Autodesk Inventor part; units mm, degrees
ref_plane "YZ Plane" through (0, 0, 0) normal (1, 0, 0) x (0, 1, 0)
ref_plane "XZ Plane" through (0, 0, 0) normal (0, 1, 0) x (-1, 0, 0)
ref_plane "XY Plane" through (0, 0, 0) normal (0, 0, 1) x (1, 0, 0)
sketch "Sketch1" plane through (0, 0, 0) normal (0, 1, 0) x (-1, 0, 0)
  circle A0 centre (0, 0) radius 13
  circle A1 centre (0, 0) radius 14.5
  dimension "d0" = 26
  dimension "d1" = 29
extrude "Extrusion1" add sketch "Sketch1" along normal blind 4
sketch "Sketch2" plane through (0, 0, 0) normal (0, -1, 0) x (1, 0, 0)
  circle A0 centre (0, 0) radius 14.5
  dimension "d4" = 29
extrude "Extrusion2" add sketch "Sketch2" along normal blind 2
sketch "Sketch3" plane through (0, 0, 0) normal (0, 1, 0) x (1, 0, 0)
  line L0 (-3.5, 3.5) -> (3.5, 3.5)
  line L1 (3.5, 3.5) -> (3.5, -3.5)
  line L2 (3.5, -3.5) -> (-3.5, -3.5)
  line L3 (-3.5, -3.5) -> (-3.5, 3.5)
  line L4 (-3.5, 3.5) -> (3.5, -3.5) construction
  line L5 (3.5, 3.5) -> (-3.5, -3.5) construction
  point P0 (0, 0)
  dimension "d7" = 7
  dimension "d8" = 7
extrude "Extrusion3" cut sketch "Sketch3" against normal blind 3
fillet "Fillet1" radius 2 1 edges at (-14.5, -2, 0)
fillet "Fillet2" radius 1 1 edges at (13, 4, 0)
sketch "Sketch4" plane through (0, 0, 0) normal (0, 1, 0) x (1, 0, 0)
  line L0 (0, 0) -> (0, -8)
  line L1 (0, 0) -> (0, 8)
  line L2 (0, 8) -> (16, 8)
  line L3 (16, 8) -> (16, 16)
  line L4 (0, 8) -> (0, 12)
  line L5 (0, 8) -> (4, 8) construction
  line L6 (-16, 16) -> (16, 16)
  line L7 (16, 16) -> (16, 8)
  line L8 (16, 8) -> (-16, 8)
  line L9 (-16, 8) -> (-16, 16)
  line L10 (-16, 16) -> (16, 8) construction
  line L11 (16, 16) -> (-16, 8) construction
  line L12 (0, -8) -> (0, -12)
  line L13 (-16, -8) -> (16, -8)
  line L14 (16, -8) -> (16, -16)
  line L15 (16, -16) -> (-16, -16)
  line L16 (-16, -16) -> (-16, -8)
  line L17 (-16, -8) -> (16, -16) construction
  line L18 (16, -8) -> (-16, -16) construction
  dimension "d13" = 8
  dimension "d14" = 8
  dimension "d15" = 16
  dimension "d16" = 8
  dimension "d17" = 4
  dimension "d18" = 90
  dimension "d19" = 4
  dimension "d20" = 32
  dimension "d21" = 8
extrude "Extrusion4" cut sketch "Sketch4" along normal mid plane 20
properties part number "Battery_Holder"
For this review, take the finished solid that the model builds, in its own axes (mm). A direction names the side the tool comes from. Coordinates: 2 decimals unless noted, no trailing zeros. Write each loop counter-clockwise with the first axis right and the second up, starting at its lowest first coordinate (ties: lowest second). Pieces come first, ordered by that corner, then holes. Notation, with made-up numbers: (79.25, 80.25) - (106.25, 80.25) arc R14 ccw to (106.25, 92.25) - close; hole circle Ø6 at (43, 7.5). An arc over 180 degrees is marked (long way). Answer in a Markdown table with one row per item. Add a question column.
Q1. Tool access review of faces 1 (the flat face through (3.5, -1, 0)), 2 (the flat face through (0, 0, 4)), 3 (the flat face through (0, -2, 4)): name each direction out of +Z, -Z, +X, -X, +Y, -Y from which nothing blocks a thin tool from reaching the whole face with its end or side.
Q2. We need section A-A, the plane x = 0. State the section outline as (y, z) points.
Q3. We need section B-B, the plane y = 1.5. State the section outline as (x, z) points.
Q4. Draft analysis for pull direction Z (two halves, no side actions). For faces 4 (the flat face through (0.2, -0.4, -8)), 5 (the cylindrical face through (14.5, 2, 0.1)), 6 (the cylindrical face through (13, 1, 0)), state which applies: +Z half, -Z half, draft (parallel to the pull), parting line (faces both ways), or undercut.
Q5. For probe 1 along Z at (x, y) = (-1, -1); probe 2 along X at (y, z) = (3.5, 2); probe 3 along X at (y, z) = (3.75, 2), list the stretches that pass through material, from the lowest coordinate up.
Q6. We need section C-C, the plane y = -0.75. State the section outline as (x, z) points, and give its area (3 significant figures).
Q7. We need section D-D, the plane x = 7.5. State the section outline as (y, z) points.
Q8. For P1, Ø1.6, axis at y = -1, z = 1, coming from the -X side; P2, Ø5, axis at x = -4, z = 0, coming from the +Y side, all flat-tipped, find the tip position at first contact; note any pin that passes through.
Answer list:
| question | item | result |
|---|---|---|
| 1 | face 1 | +Y, -Y |
| 1 | face 2 | +Y |
| 1 | face 3 | +Z, -Z, +X, -X, -Y |
| 2 | outline | (-2, -8) - (0, -8) - (0, -3.5) - (-2, -3.5) - close; (-2, 3.5) - (0, 3.5) - (0, 8) - (-2, 8) - close |
| 3 | outline | (-12.09, -8) - (-10.25, -8) arc R13 cw to (-10.25, 8) - (-12.09, 8) arc R14.5 ccw to start; (10.25, -8) - (12.09, -8) arc R14.5 ccw to (12.09, 8) - (10.25, 8) arc R13 cw to start |
| 4 | face 4 | -Z half |
| 4 | face 5 | parting line |
| 4 | face 6 | undercut |
| 5 | probe 1 | z = -8 to -3.5, 3.5 to 8 |
| 5 | probe 2 | x = -14.36 to -12.98, 12.98 to 14.36 |
| 5 | probe 3 | x = -14.36 to -13.19, 13.19 to 14.36 |
| 6 | outline | (-11.92, -8) - (11.92, -8) arc R14.35 ccw to (11.92, 8) - (-11.92, 8) arc R14.35 ccw to start; hole (-3.5, -3.5) - (3.5, -3.5) - (3.5, 3.5) - (-3.5, 3.5) - close |
| 6 | area | 385 mm2 |
| 7 | outline | (-2, -8) - (0, -8) - (0, 8) - (-2, 8) - close |
| 8 | P1 | stops at x = -14.47 |
| 8 | P2 | stops at y = 0 |
